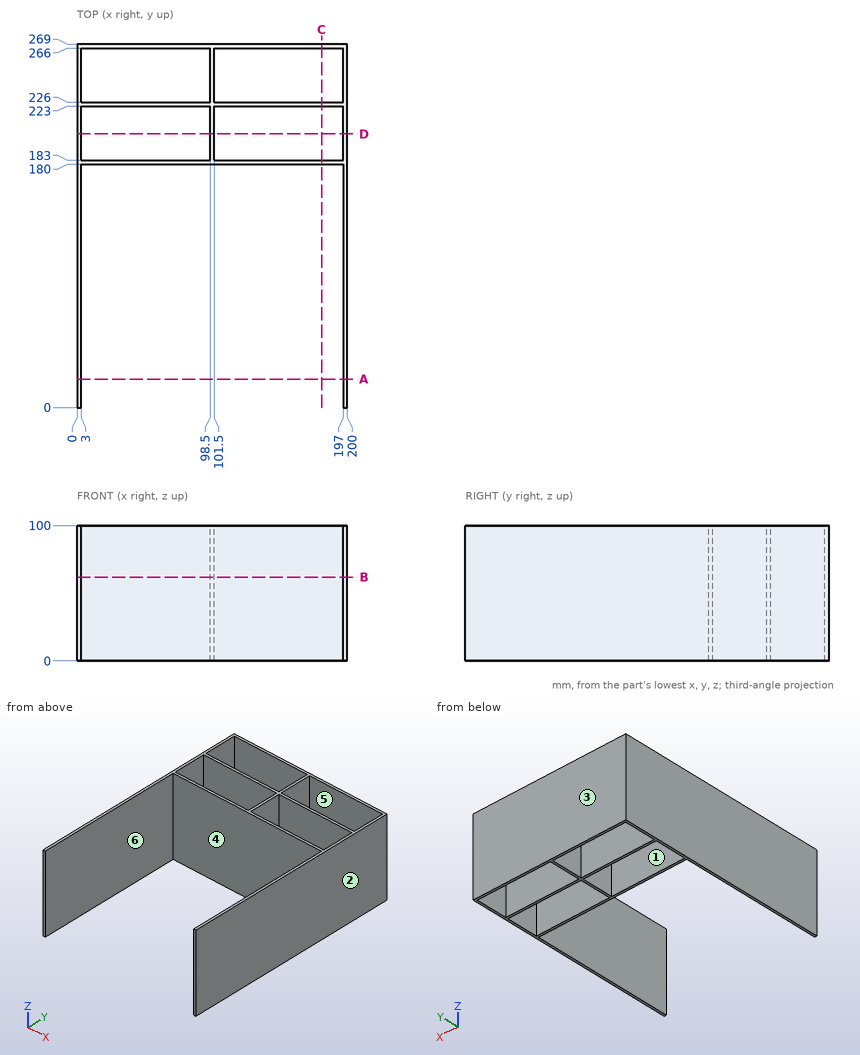
Can you work these out from the drawing? Everything is in mm from the part's minimum corner. A direction names the side the tool comes from. Round coordinates to 2 decimals unless told otherwise and drop trailing zeros. Order: outer loops, then holes, each group sorted by start corner. A loop starts at its lowest first (then second) coordinate and runs counter-clockwise, first axis right, second up.
(1) If we section it at B-B (z = 62): Please give me the cut outline in (x, y).
Results are:
outline: (0, 0) - (3, 0) - (3, 180) - (197, 180) - (197, 0) - (200, 0) - (200, 269) - (0, 269) - close; hole (3, 183) - (98.5, 183) - (98.5, 223) - (3, 223) - close; hole (3, 226) - (98.5, 226) - (98.5, 266) - (3, 266) - close; hole (101.5, 183) - (197, 183) - (197, 223) - (101.5, 223) - close; hole (101.5, 226) - (197, 226) - (197, 266) - (101.5, 266) - close
(2) If we section it at C-C (x = 181): Please give me the cut outline in (y, z).
Results are:
outline: (180, 0) - (183, 0) - (183, 100) - (180, 100) - close; (223, 0) - (226, 0) - (226, 100) - (223, 100) - close; (266, 0) - (269, 0) - (269, 100) - (266, 100) - close
(3) If we section it at D-D (y = 202.5): Please give me the cut outline in (x, z), plus the area to 3 significant figures.
Results are:
outline: (0, 0) - (3, 0) - (3, 100) - (0, 100) - close; (98.5, 0) - (101.5, 0) - (101.5, 100) - (98.5, 100) - close; (197, 0) - (200, 0) - (200, 100) - (197, 100) - close
area: 900 mm2
(4) On a 3-axis mill with a long thin cutter (end or side, diameter ignored), from which of +Z, -Z, +X, -X, +Y, -Y can I reach the whole of each face in a straight line? I mean the marked faces 5 and 6. Say none if no direction works.
Results are:
face 5: +Z, -Z
face 6: +Z, -Z, -Y
(5) We'd pull the mould along Y, two halves only. Please class the marked faces 1, 2, 3 and 4: +Y half, -Y half, draft (parallel to the pull), parting line (faces both ways), or undercut.
Results are:
face 1: undercut
face 2: draft
face 3: +Y half
face 4: -Y half
(6) I'm going to push flat-ended pins straight in: pin 1 (3 mm diameter, centred on x = 30.5, z = 56, fed in from -Y); pin 2 (6 mm diameter, centred on y = 207, z = 67.5, fed in from -X). Where does each tip first touch, or does it pass through?
Results are:
pin 1: stops at y = 180
pin 2: stops at x = 0
(7) If I drill on L1, parallel to X at y = 236, z = 55.5; L2, parallel to Y at x = 189, z = 9; L3, parallel to X at y = 89.5, z = 96.5, over which ranges is the centre line in solid material (lowest first)?
Results are:
L1: x = 0 to 3, 98.5 to 101.5, 197 to 200
L2: y = 180 to 183, 223 to 226, 266 to 269
L3: x = 0 to 3, 197 to 200
(8) If we section it at A-A (y = 21): Please give me the cut outline in (x, z), plus the area to 3 significant figures.
Results are:
outline: (0, 0) - (3, 0) - (3, 100) - (0, 100) - close; (197, 0) - (200, 0) - (200, 100) - (197, 100) - close
area: 600 mm2
